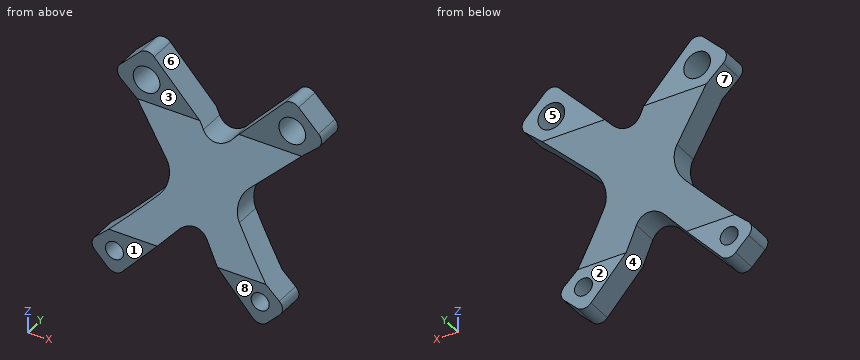
from build123d import *

# Parameters (mm, degrees)
BOSS_EXTRUDE1_DEPTH      = 4
BOSS_EXTRUDE1_DEPTH_BACK = 4
SKETCH1_R                = 1.375
SKETCH1_R_2              = 0.925
CUT_EXTRUDE1_DEPTH       = 29.461459085
CUT_EXTRUDE1_DEPTH_BACK  = 29.461459085
FILLET1_R                = 2
FILLET2_R                = 1


with BuildPart() as part:
    # Sketch1 → Boss-Extrude1 (new, two sides: drawn at the far end of the back side and taken through both)
    with BuildSketch(Plane(origin=(0, 0, 0), x_dir=(1, 0, 0), z_dir=(0, 1, 0)).offset(-BOSS_EXTRUDE1_DEPTH_BACK)):
        with BuildLine():
            ThreePointArc((-2.75, 0), (-6.398566018, 3.816356305), (-10.253048327, 7.424621202))
            Line((-10.253048327, 7.424621202), (-7.424621202, 10.253048327))
            Line((-7.424621202, 10.253048327), (0, 2))
            Line((0, 2), (0, 0))
            Line((0, 0), (0, -3))
            Line((0, -3), (-7.424621202, -10.960155108))
            Line((-7.424621202, -10.960155108), (-10.960155108, -7.424621202))
            Line((-10.960155108, -7.424621202), (-2.75, 0))
        make_face()
        with Locations(Location((-7.5, -7.5, 0), (0, 0, 270))):
            Circle(SKETCH1_R, mode=Mode.SUBTRACT)
        with Locations(Location((-7.5, 7.5, 0), (0, 0, 270))):
            Circle(SKETCH1_R_2, mode=Mode.SUBTRACT)
    extrude(amount=BOSS_EXTRUDE1_DEPTH + BOSS_EXTRUDE1_DEPTH_BACK)

    # Mirror2: part across plane


with BuildPart() as part_1:
    add(part.part)
    add(part.part.mirror(Plane(origin=(0, -4, 0), x_dir=(0, 0, 1), z_dir=(-1, 0, 0))))

    # Sketch3 → Cut-Extrude1 (cut, two sides: drawn at the far end of the back side and taken through both)
    with BuildSketch(Plane(origin=(-15, 0, 0), x_dir=(0, 0, -1), z_dir=(1, 0, 0)).offset(-CUT_EXTRUDE1_DEPTH_BACK)):
        Polygon((5.45, -1.3), (10.25, -1.3), (10.25, 4), (-5.16, 4), align=None)
        Polygon((-10.96, -4), (5.45, -4), (-5.16, 1.3), (-10.96, 1.3), align=None)
    extrude(amount=CUT_EXTRUDE1_DEPTH + CUT_EXTRUDE1_DEPTH_BACK, mode=Mode.SUBTRACT)

    # Fillet1
    fillet1_edges = [part_1.edges().sort_by_distance(p)[0] for p in [
        (2.75, 0.072431668, 0),
        (-2.75, 0.072431668, 0),
        (0, -0.926625825, -2),
        (0, 1.571017908, 3),
    ]]
    fillet(fillet1_edges, radius=FILLET1_R)

    # Fillet2
    fillet2_edges = [part_1.edges().sort_by_distance(p)[0] for p in [
        (-7.424621202, 0, -10.253048327),
        (-10.253048327, -2.65, -7.424621202),
        (7.424621202, 0, -10.253048327),
        (10.253048327, -2.65, -7.424621202),
        (10.960155108, 2.65, 7.424621202),
        (7.424621202, 0, 10.960155108),
        (-10.960155108, 2.65, 7.424621202),
        (-7.424621202, 0, 10.960155108),
    ]]
    fillet(fillet2_edges, radius=FILLET2_R)


solid = part_1.part
For this review, take the finished solid that the model builds, in its own axes (mm). Face numbers are marked on the shaded views. A direction names the side the tool comes from. Give positions to 0.01 mm unless a question says otherwise; leave off trailing zeros. Loops run counter-clockwise (first coordinate to the right, second up) from the corner with the lowest first, then second, coordinate; pieces in that order, holes last.
Item 1: Insertion check: pin 1 (4.5 mm diameter, centred on x = 7, z = 8.5, fed in from -Y); pin 2 (2 mm diameter, centred on x = -4.5, z = -4, fed in from -Y); pin 3 (2 mm diameter, centred on y = 0, z = -2, fed in from -X). Each pin has a flat end and moves straight along its axis. Give the tip position at first contact, or say it passes through.
Item 2: Take a section at D-D, the plane z = 7.5. State the section outline as (x, y) points (3 decimals), and give its area (3 significant figures).
Item 3: For line 1 along Y through (x, z) = (4.75, -7); line 2 along X through (y, z) = (-0.5, -0.25); line 3 along X through (y, z) = (1.75, 4.75), list the stretches that pass through material, from the lowest coordinate up.
Item 4: Take a section at C-C, the plane x = 7.5. State the section outline as (y, z) points (3 decimals), and give its area (3 significant figures).
Item 5: Draft analysis for pull direction X (two halves, no side actions). For the marked faces 5, 6, 7 and 8, state which applies: +X half, -X half, draft (parallel to the pull), parting line (faces both ways), or undercut.
Item 6: Take a section at A-A, the plane z = -7.5. State the section outline as (x, y) points (3 decimals), and give its area (3 significant figures).
Item 7: Take a section at B-B, the plane y = 3.25. State the section outline as (x, z) points (3 decimals), and give its area (3 significant figures).
Item 8: Tool access review of the marked faces 1, 2, 3 and 4: name each direction out of +Z, -Z, +X, -X, +Y, -Y from which nothing blocks a thin tool from reaching the whole face with its end or side.
Calculated:
1. pin 1: stops at y = 1.3
1. pin 2: stops at y = -3.78
1. pin 3: stops at x = -5.58
2. outline: (-10.509, 1.3) - (-8.875, 1.3) - (-8.875, 4) - (-10.509, 4) - close; (-6.125, 1.3) - (-4.197, 1.3) - (-4.197, 4) - (-6.125, 4) - close; (4.197, 1.3) - (6.125, 1.3) - (6.125, 4) - (4.197, 4) - close; (8.875, 1.3) - (10.509, 1.3) - (10.509, 4) - (8.875, 4) - close
2. area: 19.2 mm2
3. line 1: y = -4 to -1.3
3. line 2: x = -3.59 to 3.59
3. line 3: x = -8 to -1.63, 1.63 to 8
4. outline: (-4, -9.8) - (-1.3, -9.8) - (-1.3, -8.425) - (-4, -8.425) - close; (-4, -6.575) - (-1.3, -6.575) - (-1.3, -5.45) - (-1.02, -4.889) - (-3.72, -4.889) - (-4, -5.45) - close; (0.868, 4.296) - (3.568, 4.296) - (4, 5.16) - (4, 6.125) - (1.3, 6.125) - (1.3, 5.16) - close; (1.3, 8.875) - (4, 8.875) - (4, 10.52) - (1.3, 10.52) - close
4. area: 17.6 mm2
5. face 5: undercut
5. face 6: undercut
5. face 7: -X half
5. face 8: draft
6. outline: (-9.798, -4) - (-8.425, -4) - (-8.425, -1.3) - (-9.798, -1.3) - close; (-6.575, -4) - (-4.948, -4) - (-4.948, -1.3) - (-6.575, -1.3) - close; (4.948, -4) - (6.575, -4) - (6.575, -1.3) - (4.948, -1.3) - close; (8.425, -4) - (9.798, -4) - (9.798, -1.3) - (8.425, -1.3) - close
6. area: 16.2 mm2
7. outline: (-10.217, 8.168) arc R1 ccw to (-10.18, 6.719) - (-6.796, 3.659) - (6.796, 3.659) - (10.18, 6.719) arc R1 ccw to (10.217, 8.168) - (8.157, 10.228) arc R1 ccw to (6.718, 10.203) - (1.463, 4.568) arc R2 cw to (-1.463, 4.568) - (-6.718, 10.203) arc R1 ccw to (-8.157, 10.228) - close; hole circle Ø2.75 at (-7.5, 7.5); hole circle Ø2.75 at (7.5, 7.5)
7. area: 60.9 mm2
8. face 1: +Z, -Z, +X, -X, -Y
8. face 2: -Z, +X, -X, +Y
8. face 3: +Z, +X, -X, -Y
8. face 4: -Z, +Y, -Y
